The listing builds one solid part. Answer for the finished solid, in the listing's coordinates (mm). Face numbers are marked on the shaded views. A direction names the side the tool comes from. Give positions to 0.01 mm unless a question says otherwise; leave off trailing zeros. Loops run counter-clockwise (first coordinate to the right, second up) from the corner with the lowest first, then second, coordinate; pieces in that order, holes last. Notation, with made-up numbers: (-13, 24.5) - (7, 24.5) arc R30 ccw to (7, 63.5) - close; hole circle Ø8 at (59.25, 57). An arc over 180 degrees is marked (long way). Answer as CSV lines item,"result". Start each with the question number.
1) A cutting plane is placed at A-A (z = -25.4). Determine the outline of the cut face in (x, y) (3 decimals), and give its area (3 significant figures).
2) Flat-ended cylindrical pins translate along their axes: pin 1 (6.5 mm diameter, centred on x = 38.1, y = 69.85, fed in from -Z) (3 decimals); pin 2 (1.5 mm diameter, centred on x = -4.5, z = -42.5, fed in from +Y) (3 decimals); pin 3 (1 mm diameter, centred on x = 8, y = 8.5, fed in from -Z). Find the tip coordinate at first contact, or state that the pin passes through.
3) For the marked faces 1 and 2, determine the directions among +Z, -Z, +X, -X, +Y, -Y from which every point of the face is accessible in a straight line to the end or side of a thin tool.
4) Find the intervals of material crossed by line 1 along X through (y, z) = (5.75, -25.4) (3 decimals); line 2 along X through (y, z) = (2.75, -50.8) (3 decimals); line 3 along Z through (x, y) = (38.1, 3.75), in increasing order.
5) A cutting plane is placed at B-B (x = -12.7). Determine the outline of the cut face in (y, z) (3 decimals), and give its area (3 significant figures).
6) A cutting plane is placed at C-C (y = 69.85). Determine the outline of the cut face in (x, z) (3 decimals), and give its area (3 significant figures).
7) A cutting plane is placed at D-D (x = -38.1). Determine the outline of the cut face in (y, z) (3 decimals), and give its area (3 significant figures).
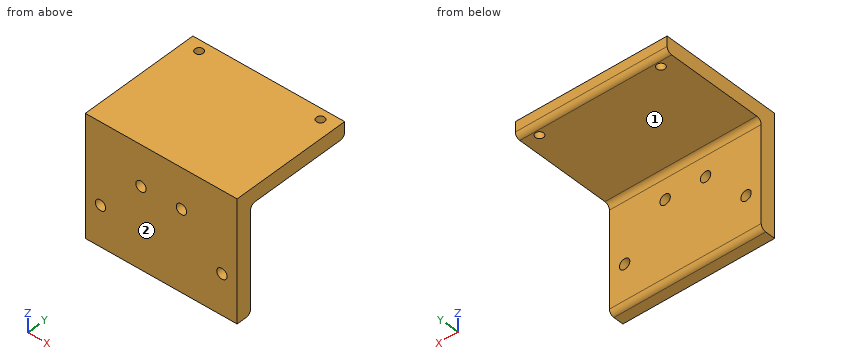
```python
from build123d import *

# Parameters (mm, degrees)
BOSS_EXTRUDE1_DEPTH     = 47.625
FILLET1_R               = 3.175
F_1_4_20_TAPPED_HOLE1_D = 5.1054
F_1_4_CLEARANCE_HOLE1_D = 6.5278


with BuildPart() as part:
    # Sketch1 → Boss-Extrude1 (new, symmetric)
    with BuildSketch(Plane(origin=(0, 0, 0), x_dir=(0, 0, -1), z_dir=(1, 0, 0))):
        Polygon((0, 76.2), (0, 0), (76.2, 0), (76.2, 9.525), (9.525, 9.525), (9.525, 76.2), align=None)
    extrude(amount=BOSS_EXTRUDE1_DEPTH, both=True)

    # Fillet1
    fillet1_edges = [part.edges().sort_by_distance(p)[0] for p in [
        (0, 76.2, -9.525),
        (0, 9.525, -9.525),
        (0, 9.525, -76.2),
    ]]
    fillet(fillet1_edges, radius=FILLET1_R)

    # 1/4-20 Tapped Hole1 (through all)
    with Locations(Plane.XY):
        with Locations((-38.1, 69.85), (38.1, 69.85)):
            Hole(F_1_4_20_TAPPED_HOLE1_D / 2)

    # 1/4 Clearance Hole1 (through all)
    with Locations(Plane(origin=(0, 9.525, 0), x_dir=(1, 0, 0), z_dir=(0, 1, 0))):
        with Locations((-38.1, 50.8), (38.1, 50.8), (-12.7, 25.4), (12.7, 25.4)):
            Hole(F_1_4_CLEARANCE_HOLE1_D / 2)


solid = part.part
```
Ans:
1,outline,"(-47.625, 0) - (-15.964, 0) - (-15.964, 9.525) - (-47.625, 9.525) - close; (-9.436, 0) - (9.436, 0) - (9.436, 9.525) - (-9.436, 9.525) - close; (15.964, 0) - (47.625, 0) - (47.625, 9.525) - (15.964, 9.525) - close"
1,area,"783 mm2"
2,pin 1,"z = -9.525"
2,pin 2,"y = 9.525"
2,pin 3,"z = -75.74"
3,face 1,"-Z, +X, -X, +Y"
3,face 2,"+Z, -Z, +X, -X, -Y"
4,line 1,"-47.625 to -15.964, -9.436 to 9.436, 15.964 to 47.625"
4,line 2,"-47.625 to -41.364, -34.836 to 34.836, 41.364 to 47.625"
4,line 3,"-76.2 to -54.06, -47.54 to 0"
5,outline,"(0, -76.2) - (6.35, -76.2) arc R3.175 ccw to (9.525, -73.025) - (9.525, -28.664) - (0, -28.664) - close; (0, -22.136) - (9.525, -22.136) - (9.525, -12.7) arc R3.175 cw to (12.7, -9.525) - (73.025, -9.525) arc R3.175 ccw to (76.2, -6.35) - (76.2, 0) - (0, 0) - close"
5,area,"1,300 mm2"
6,outline,"(-47.625, -9.525) - (-40.653, -9.525) - (-40.653, 0) - (-47.625, 0) - close; (-35.547, -9.525) - (35.547, -9.525) - (35.547, 0) - (-35.547, 0) - close; (40.653, -9.525) - (47.625, -9.525) - (47.625, 0) - (40.653, 0) - close"
6,area,"810 mm2"
7,outline,"(0, -76.2) - (6.35, -76.2) arc R3.175 ccw to (9.525, -73.025) - (9.525, -54.064) - (0, -54.064) - close; (0, -47.536) - (9.525, -47.536) - (9.525, -12.7) arc R3.175 cw to (12.7, -9.525) - (67.297, -9.525) - (67.297, 0) - (0, 0) - close; (72.403, -9.525) - (73.025, -9.525) arc R3.175 ccw to (76.2, -6.35) - (76.2, 0) - (72.403, 0) - close"
7,area,"1,250 mm2"
